Design review of the part built by this model. Coordinates are the model's own, in mm. A direction names the side the tool comes from. Round coordinates to 2 decimals unless told otherwise and drop trailing zeros. Write each loop counter-clockwise with the first axis right and the second up, starting at its lowest first coordinate (ties: lowest second). Pieces come first, ordered by that corner, then holes. Notation, with made-up numbers: (8, -19) -> (50, -19) arc R22 ccw to (50, 15) -> close; hole circle Ø11 at (-32.5, 5). An arc over 180 degrees is marked (long way). Write item = value, one per line. Start each with the question number.
Item 1: Machinability: for faces 5 (the flat face through (29.72, -99.26, 45.865)), 6 (the flat face through (79, -84, 2.5)), 7 (the flat face through (61, -100, 28)), which of the approach directions +Z, -Z, +X, -X, +Y, -Y give a long, thin tool a straight path to every point of the face, cutting with its end or side? Answer none if there is none.
Item 2: Add section A-A, the plane z = 71. State the section outline as (x, y) points, then the cut area to 3 significant figures.
Item 3: For pin 1 Ø4 at (x, z) = (107.5, 70) entering from -Y, flat-tipped, find the tip position at first contact; note if it passes through.
Item 4: Add section B-B, the plane x = 41. State the section outline as (y, z) points.
Item 5: To check wall thickness, follow L1, parallel to Y at x = 49, z = 36; L2, parallel to Z at x = 84.5, y = -75; L3, parallel to Y at x = 149, z = 51. State the ranges of each line that lie inside material, in increasing order.
Item 6: Mouldability with a two-part tool opening along X and no side actions: class faces 1 (the flat face through (0, -49, 49)), 2 (the flat face through (79, -49, 0)), 3 (the cylindrical face through (68.1, -99.3, 29.1)), 4 (the flat face through (160, -49, 49)) as released by +X, released by -X, zero draft, split by the parting line, or undercut.
from build123d import *

# Parameters (mm, degrees)
F0_W     = 160
F0_H     = 100
F1_DEPTH = 100
F3_DEPTH = 50
F4_T     = -2.5
F5_W     = 155
F5_H     = 95
F6_DEPTH = 67.5
F8_W     = 150
F8_H     = 90
F9_DEPTH = 1
F10_R    = 2


with BuildPart() as f1:
    # F0 (on Front) → F1 (new body)
    with BuildSketch(Plane.XZ):
        with Locations((80, 50)):
            Rectangle(F0_W, F0_H)
    extrude(amount=F1_DEPTH)

    # F2 (on face) → F3 (cut)
    with BuildSketch(Plane.XZ.offset(100)):
        with BuildLine():
            Line((141, 10), (141, 50))
            Line((141, 50), (141, 92.5))
            Line((141, 92.5), (10, 92.5))
            Line((10, 92.5), (10, 57.5))
            Line((10, 57.5), (50, 33.9))
            ThreePointArc((50, 33.9), (68.2476049495, 28.8997849974), (67.3670576668, 10))
            Line((67.3670576668, 10), (80, 10))
            Line((80, 10), (141, 10))
        make_face()
    extrude(amount=-F3_DEPTH, mode=Mode.SUBTRACT)

    # F4
    f4_openings = [f1.faces().sort_by_distance(p)[0] for p in [
        (10, -75, 75),
        (30, -75, 45.7),
        (68.247605, -75, 28.899785),
        (104.183529, -75, 10),
        (141, -75, 51.25),
        (83.977871, -50, 56.442025),
        (75.5, -75, 92.5),
    ]]
    offset(amount=F4_T, openings=f4_openings)

    # F5 (on face) → F6 (join)
    with BuildSketch(Plane.XZ.offset(2.5)):
        with Locations((80, 50)):
            Rectangle(F5_W, F5_H)
    extrude(amount=F6_DEPTH)

    # F8 (on offset) → F9 (join)
    with BuildSketch(Plane.XZ.offset(97.5)):
        with Locations((80, 50)):
            Rectangle(F8_W, F8_H)
    extrude(amount=F9_DEPTH)

    # F10
    f10_edges = [f1.edges().sort_by_distance(p)[0] for p in [
        (10, -99.25, 92.5),
        (141, -99.25, 92.5),
        (141, -99.25, 10),
    ]]
    fillet(f10_edges, radius=F10_R)


solid = f1.part
Result set:
q1.face_5 = -Y
q1.face_6 = none
q1.face_7 = +Z, -Z, +X, -X, -Y
q2.outline = (0, -100) -> (10, -100) -> (10, -98.5) -> (141, -98.5) -> (141, -100) -> (160, -100) -> (160, 0) -> (0, 0) -> close; hole (2.5, -97.5) -> (157.5, -97.5) -> (157.5, -70) -> (2.5, -70) -> close
q2.area = 11,500 mm²
q3.pin_1 = -98.5
q4.outline = (-100, 0) -> (0, 0) -> (0, 100) -> (-100, 100) -> (-100, 92.5) -> (-98.5, 92.5) -> (-98.5, 39.21) -> (-100, 39.21) -> close; hole (-97.5, 2.5) -> (-70, 2.5) -> (-70, 97.5) -> (-97.5, 97.5) -> close
q5.L1 = -98.5 to -97.5, -70 to 0
q5.L2 = 0 to 2.5, 97.5 to 100
q5.L3 = -100 to -97.5, -70 to 0
q6.face_1 = released by -X
q6.face_2 = zero draft
q6.face_3 = undercut
q6.face_4 = released by +X
